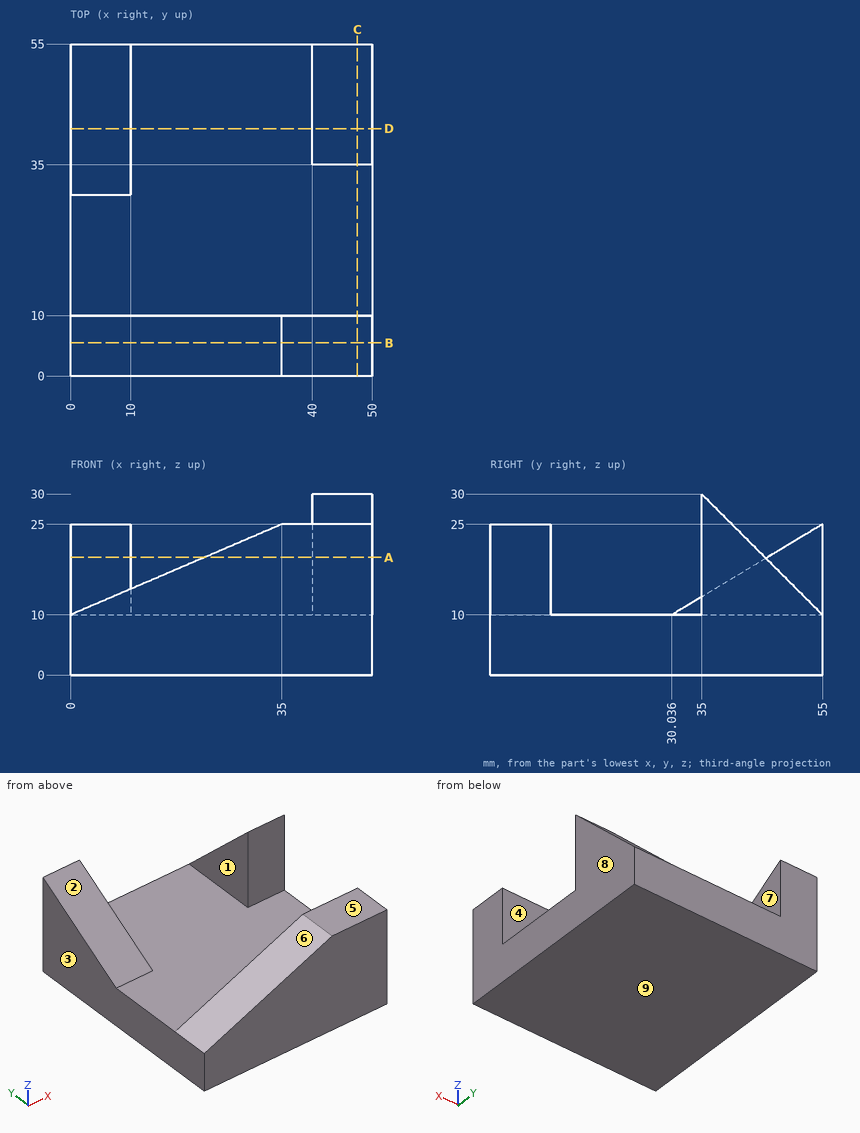
Could you check a few things on this drawing? It's one solid part, dimensions in mm from its lowest x, y, z. A direction names the side the tool comes from. Coordinates: 2 decimals unless noted, no trailing zeros. Order: outer loops, then holes, each group sorted by start corner. A loop starts at its lowest first (then second) coordinate and runs counter-clockwise, first axis right, second up. Notation, with made-up numbers: M 3,79.25 L 55,79.25 A24 cw 55,115.25 Z; hole C 19,62 d4. An arc over 180 degrees is marked long. Use a Markdown table: item, result. Add a question column.
Q1. I want a section at C-C on x = 47.5. List the corners of the cut face in (y, z) for me.
Q2. I want a section at B-B on y = 5.5. List the corners of the cut face in (x, z) for me, then the cut area to 4 significant figures.
Q3. I'm going to push flat-ended pins straight in: pin 1 (2 mm diameter, centred on x = 43.5, y = 25.5, fed in from +Z); pin 2 (7.5 mm diameter, centred on x = 21.5, z = 14.5, fed in from +Y); pin 3 (3 mm diameter, centred on x = 43.5, y = 39.5, fed in from +Z). Where does each tip first touch, or does it pass through?
Q4. I want a section at A-A on z = 19.5. List the corners of the cut face in (x, y) for me.
Q5. Which directions (+Z, -Z, +X, -X, +Y, -Y) give clear straight access to the entire face, cutting with the end or side of a thin tool? Please do the marked faces 1, 2, 3, 4 and 5.
Q6. I want a section at D-D on y = 41. List the corners of the cut face in (x, z) for me.
Q7. We'd pull the mould along X, two halves only. Please class the marked faces 6, 7, 8 and 9: pulls with the +X half, pulls with the -X half, needs draft (parallel to the pull), parting line crosses it, or undercut.
Q8. If I drill on L1, parallel to X at y = 39, z = 10.5; L2, parallel to X at y = 42.5, z = 21.5; L3, parallel to Z at x = 9.5, y = 28.5, over which ranges is the centre line in solid material (lowest first)?
Checked values:
| question | item | result |
|---|---|---|
| 1 | outline | M 0,0 L 55,0 L 55,10 L 35,30 L 35,10 L 10,10 L 10,25 L 0,25 Z |
| 2 | outline | M 0,0 L 50,0 L 50,25 L 35,25 L 0,10 Z |
| 2 | area | 987.5 mm² |
| 3 | pin 1 | z = 10 |
| 3 | pin 2 | y = 10 |
| 3 | pin 3 | z = 27 |
| 4 | outline | M 0,45.85 L 10,45.85 L 10,55 L 0,55 Z; M 22.17,0 L 50,0 L 50,10 L 22.17,10 Z; M 40,35 L 50,35 L 50,45.5 L 40,45.5 Z |
| 5 | face 1 | +Z, +Y |
| 5 | face 2 | +Z, -X |
| 5 | face 3 | +Z, -Z, -X, +Y, -Y |
| 5 | face 4 | +Z, +X, -X |
| 5 | face 5 | +Z, +X, -X, -Y |
| 6 | outline | M 0,0 L 50,0 L 50,24 L 40,24 L 40,10 L 10,10 L 10,16.59 L 0,16.59 Z |
| 7 | face 6 | pulls with the -X half |
| 7 | face 7 | undercut |
| 7 | face 8 | pulls with the +X half |
| 7 | face 9 | needs draft |
| 8 | L1 | 0 to 10, 40 to 50 |
| 8 | L2 | 40 to 50 |
| 8 | L3 | 0 to 10 |
